Build history of the part. All positions in model axes, mm. Face numbers are marked on the shaded views. A direction names the side the tool comes from. Give positions to 0.01 mm unless a question says otherwise; leave off trailing zeros. Order: outer loops, then holes, each group sorted by start corner. A loop starts at its lowest first (then second) coordinate and runs counter-clockwise, first axis right, second up. Notation, with made-up numbers: (15, 33) - (25, 33) arc R25 ccw to (25, 45) - close; hole circle Ø3 at (-8, 78.25). An arc over 180 degrees is marked (long way). Write each question's results on one line, items separated by ' | '. Start each with the question number.
1) Tool access for the marked faces 4, 5 and 6: list every direction of +Z, -Z, +X, -X, +Y, -Y with a clear straight run to the whole face (end or side of a thin tool).
2) Cut at D-D on x = 2. List the corners of the cut face in (y, z).
3) Cut at A-A on z = 2.5. List the corners of the cut face in (x, y) (3 decimals).
4) Cut at B-B on x = 0. List the corners of the cut face in (y, z) (3 decimals), plus the area to 3 significant figures.
5) Drill centre lines: line 1 along X through (y, z) = (0, 6.5) (3 decimals); line 2 along X through (y, z) = (-3.75, 7.5). Where is each one in solid material? Low to high. Write a range as from..to.
6) Two-plate mould, pull along X, no slides. Class the marked faces 1, 2 and 3: +X half, -X half, draft (parallel to the pull), parting line (faces both ways), or undercut.
7) Drop flat-ended pins along their axis: pin 1 Ø3 at (x, y) = (-1.5, -1) entering from +Z; pin 2 Ø1.5 at (x, y) = (-4.5, -0.5) entering from +Z; pin 3 Ø1.2 at (x, y) = (-3.965, -3.965) entering from -Z; pin 4 Ø1.7 at (x, y) = (3.5, 4) entering from -Z. Give the stop position or say it passes through.
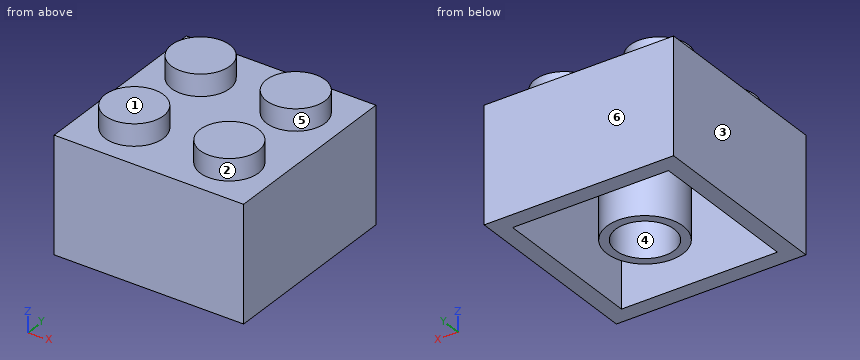
from build123d import *

# Parameters (mm, degrees)
F0_R     = 2.435
F1_DEPTH = 9.6
F2_DEPTH = 11.4
F3_T     = -1.4
F4_R     = 3.17
F4_R_2   = 2.445
F5_DEPTH = 9.5


with BuildPart() as f1:
    # F0 (on Top) → F1 (new body)
    with BuildSketch(Plane.XY):
        Polygon((7.9, 7.9), (-7.9, 7.9), (-7.9, 3.965), (-7.9, -7.9), (7.9, -7.9), align=None)
        with Locations((-3.965, -3.965)):
            Circle(F0_R, mode=Mode.SUBTRACT)
        with Locations((3.965, -3.965)):
            Circle(F0_R, mode=Mode.SUBTRACT)
        with BuildLine():
            ThreePointArc((-1.53, 3.965), (-3.965, 1.53), (-6.4, 3.965))
            ThreePointArc((-6.4, 3.965), (-3.965, 6.4), (-1.53, 3.965))
        make_face(mode=Mode.SUBTRACT)
        with BuildLine():
            ThreePointArc((6.4, 3.965), (3.965, 1.53), (1.53, 3.965))
            ThreePointArc((1.53, 3.965), (3.965, 6.4), (6.4, 3.965))
        make_face(mode=Mode.SUBTRACT)
    extrude(amount=F1_DEPTH)

    # F0 (on Top) → F2 (join)
    with BuildSketch(Plane.XY):
        with BuildLine():
            ThreePointArc((-1.53, 3.965), (-3.965, 6.4), (-6.4, 3.965))
            ThreePointArc((-6.4, 3.965), (-3.965, 1.53), (-1.53, 3.965))
        make_face()
        with BuildLine():
            ThreePointArc((6.4, 3.965), (3.965, 6.4), (1.53, 3.965))
            ThreePointArc((1.53, 3.965), (3.965, 1.53), (6.4, 3.965))
        make_face()
        with Locations((3.965, -3.965)):
            Circle(F0_R)
        with Locations((-3.965, -3.965)):
            Circle(F0_R)
    extrude(amount=F2_DEPTH)

    # F3
    f3_openings = [f1.faces().sort_by_distance(p)[0] for p in [
        (0, 0, 0),
    ]]
    offset(amount=F3_T, openings=f3_openings, kind=Kind.INTERSECTION)

    # F4 (on face) → F5 (join)
    with BuildSketch(Plane.XY):
        Circle(F4_R)
        Circle(F4_R_2, mode=Mode.SUBTRACT)
    extrude(amount=F5_DEPTH)


solid = f1.part
Results:
1) face 4: -Z | face 5: +Z | face 6: +Z, -Z, +X, -X, +Y
2) outline: (-7.9, 0) - (-6.5, 0) - (-6.5, 8.2) - (-2.46, 8.2) - (-2.46, 0) - (-1.41, 0) - (-1.41, 8.2) - (1.41, 8.2) - (1.41, 0) - (2.46, 0) - (2.46, 8.2) - (6.5, 8.2) - (6.5, 0) - (7.9, 0) - (7.9, 9.6) - (5.4, 9.6) - (5.4, 11.4) - (2.53, 11.4) - (2.53, 9.6) - (-2.53, 9.6) - (-2.53, 11.4) - (-5.4, 11.4) - (-5.4, 9.6) - (-7.9, 9.6) - close
3) outline: (-7.9, -7.9) - (7.9, -7.9) - (7.9, 7.9) - (-7.9, 7.9) - close; circle Ø6.34 at (0, 0); hole (-6.5, -6.5) - (6.5, -6.5) - (6.5, 6.5) - (-6.5, 6.5) - close; hole circle Ø4.89 at (0, 0)
4) outline: (-7.9, 0) - (-6.5, 0) - (-6.5, 8.2) - (-3.17, 8.2) - (-3.17, 0) - (-2.445, 0) - (-2.445, 8.2) - (2.445, 8.2) - (2.445, 0) - (3.17, 0) - (3.17, 8.2) - (6.5, 8.2) - (6.5, 0) - (7.9, 0) - (7.9, 9.6) - (-7.9, 9.6) - close | area: 57.0 mm^2
5) line 1: -7.9..-6.5, -3.17..-2.445, 2.445..3.17, 6.5..7.9 | line 2: -7.9..-6.5, 6.5..7.9
6) face 1: draft | face 2: undercut | face 3: -X half
7) pin 1: z = 11.4 | pin 2: z = 9.6 | pin 3: z = 10 | pin 4: z = 8.2
